Geometry check sheet. Reference: the model listing, model coordinates, mm. A direction names the side the tool comes from. Round coordinates to 2 decimals unless told otherwise and drop trailing zeros. Loops run counter-clockwise (first coordinate to the right, second up) from the corner with the lowest first, then second, coordinate; pieces in that order, holes last. Notation, with made-up numbers: (5.5, 24) - (21.5, 24) arc R31 cw to (21.5, 51) - close; hole circle Ø9 at (-2.75, 25). An arc over 180 degrees is marked (long way). Write item = value, one per line.
```python
from build123d import *

# Parameters (mm, degrees)
SKETCH1_W           = 40
SKETCH1_H           = 100
BOSS_EXTRUDE1_DEPTH = 10
SKETCH2_W           = 30
SKETCH2_H           = 30
BOSS_EXTRUDE2_DEPTH = 10
SKETCH3_R           = 10
CUT_EXTRUDE1_DEPTH  = 10


with BuildPart() as part:
    # Sketch1 → Boss-Extrude1 (new body)
    with BuildSketch(Plane(origin=(0, 0, 0), x_dir=(0, 0, -1), z_dir=(1, 0, 0))):
        Rectangle(SKETCH1_W, SKETCH1_H)
    extrude(amount=BOSS_EXTRUDE1_DEPTH)

    # Sketch2 → Boss-Extrude2 (add)
    with BuildSketch(Plane.ZY):
        Rectangle(SKETCH2_W, SKETCH2_H)
    extrude(amount=BOSS_EXTRUDE2_DEPTH)

    # Sketch3 → Cut-Extrude1 (cut)
    with BuildSketch(Plane.ZY.offset(10)):
        Circle(SKETCH3_R)
    extrude(amount=-CUT_EXTRUDE1_DEPTH, mode=Mode.SUBTRACT)


solid = part.part
```
(1) Section check A-A (y = 0). Enter the section's corners in (x, z).
Answers follow:
outline = (-10, -15) - (0, -15) - (0, -20) - (10, -20) - (10, 20) - (0, 20) - (0, 15) - (-10, 15) - (-10, 10) - (0, 10) - (0, -10) - (-10, -10) - close
(2) Mould release check, pull along Y, two halves, no side actions. Record for faces 4 (the flat face through (5, 50, 0)), 5 (the flat face through (0, 0, 0)), 6 (the flat face through (-5, 0, 15)): pulls with the +Y half, pulls with the -Y half, needs draft (parallel to the pull), parting line crosses it, or undercut.
Answers follow:
face_4 = pulls with the +Y half
face_5 = undercut
face_6 = needs draft
(3) Scan lines: L1, parallel to Y at x = -2.75, z = 0; L2, parallel to X at y = 33.5, z = -5; L3, parallel to Y at x = -5.75, z = -12.5. Record each from-to range of solid material in increasing order. Write a range as [from, to].
Answers follow:
L1 = [-15, -10], [10, 15]
L2 = [0, 10]
L3 = [-15, 15]
(4) Section check B-B (z = 0). Enter the section's corners in (x, y), then the cut area to 3 significant figures.
Answers follow:
outline = (-10, -15) - (0, -15) - (0, -50) - (10, -50) - (10, 50) - (0, 50) - (0, 15) - (-10, 15) - (-10, 10) - (0, 10) - (0, -10) - (-10, -10) - close
area = 1,100 mm²
(5) Set-up check for faces 1 (the flat face through (-5, 15, 0)), 2 (the flat face through (-5, -15, 0)), 3 (the cylindrical face through (-5.07, -9.76, -2.17)): record each of +Z, -Z, +X, -X, +Y, -Y from which the full face is reachable in a straight line by a thin tool's end or side.
Answers follow:
face_1 = +Z, -Z, -X, +Y
face_2 = +Z, -Z, -X, -Y
face_3 = -X
(6) Gauge pin test, flat ends, axial feed: pin 1 (3 mm diameter, centred on x = -4, y = 5, fed in from -Z); pin 2 (3 mm diameter, centred on x = -6, y = -1, fed in from +Z); pin 3 (1.5 mm diameter, centred on x = -7, z = 15.5, fed in from -Y). Record the tip position at first contact, or that the pin passes through.
Answers follow:
pin_1 = -15
pin_2 = 15
pin_3 = -15
(7) Section check C-C (z = -16). Enter the section's corners in (x, y), then the cut area to 3 significant figures.
Answers follow:
outline = (0, -50) - (10, -50) - (10, 50) - (0, 50) - close
area = 1,000 mm²
(8) Section check D-D (y = -37). Enter the section's corners in (x, z), then the cut area to 3 significant figures.
Answers follow:
outline = (0, -20) - (10, -20) - (10, 20) - (0, 20) - close
area = 400 mm²
